from build123d import *

# Parameters (mm, degrees)
SKETCH004_R     = 64.00438
PAD_DEPTH       = 20
SKETCH006_R     = 4.5
POCKET_DEPTH    = 20
SKETCH005_R     = 4.5
POCKET001_DEPTH = 20
SKETCH007_W     = 10
SKETCH007_H     = 22
PAD001_DEPTH    = 70
SKETCH_W        = 16
SKETCH_H        = 40.7
POCKET002_DEPTH = 10
POCKET003_DEPTH = 20
SKETCH008_R     = 15
POCKET004_DEPTH = 20
SKETCH011_R     = 15
POCKET005_DEPTH = 20


with BuildPart() as part:
    # Sketch004 → Pad (new body)
    with BuildSketch(Plane.XY):
        Circle(SKETCH004_R)
    extrude(amount=PAD_DEPTH)

    # Sketch006 → Pocket (cut)
    with BuildSketch(Plane.XY):
        with Locations((20, 0)):
            Circle(SKETCH006_R)
    extrude(amount=POCKET_DEPTH, mode=Mode.SUBTRACT)

    # Sketch005 → Pocket001 (cut)
    with BuildSketch(Plane.XY):
        with Locations((-20, 0)):
            Circle(SKETCH005_R)
    extrude(amount=POCKET001_DEPTH, mode=Mode.SUBTRACT)

    # Sketch007 → Pad001 (join)
    with BuildSketch(Plane.XY):
        with Locations((-8, 0)):
            Rectangle(SKETCH007_W, SKETCH007_H)
    extrude(amount=-PAD001_DEPTH)

    # Sketch (on Face7 of Pad001) → Pocket002 (cut)
    with BuildSketch(Plane.YZ.offset(-3)):
        with Locations((0, -41.65)):
            Rectangle(SKETCH_W, SKETCH_H)
    extrude(amount=-POCKET002_DEPTH, mode=Mode.SUBTRACT)

    # Sketch001 → Pocket003 (cut)
    with BuildSketch(Plane.XY):
        with BuildLine():
            Line((-2.25, 1.75), (2.25, 1.75))
            ThreePointArc((2.25, -1.75), (2.850439, 0), (2.25, 1.75))
            Line((-2.25, -1.75), (2.25, -1.75))
            ThreePointArc((-2.25, 1.75), (-2.850439, 0), (-2.25, -1.75))
        make_face()
    extrude(amount=POCKET003_DEPTH, mode=Mode.SUBTRACT)

    # Sketch008 → Pocket004 (cut)
    with BuildSketch(Plane.XY):
        with Locations((0, 32)):
            Circle(SKETCH008_R)
    extrude(amount=POCKET004_DEPTH, mode=Mode.SUBTRACT)

    # Sketch011 → Pocket005 (cut)
    with BuildSketch(Plane.XY):
        with Locations((0, -32)):
            Circle(SKETCH011_R)
    extrude(amount=POCKET005_DEPTH, mode=Mode.SUBTRACT)


solid = part.part
Design review of the part built by this model. Coordinates are the model's own, in mm. A direction names the side the tool comes from. Coordinates: 2 decimals unless noted, no trailing zeros. Order: outer loops, then holes, each group sorted by start corner. A loop starts at its lowest first (then second) coordinate and runs counter-clockwise, first axis right, second up. Notation, with made-up numbers: (-4, -20.5) -> (1, -20.5) arc R35 cw to (1, 12.5) -> close; hole circle Ø2 at (75.25, 34.25). An arc over 180 degrees is marked (long way). One line per item, written item: value.
1) To check wall thickness, follow probe 1 along Y at (x, z) = (0, 14); probe 2 along Z at (x, y) = (-23, -24.5); probe 3 along Y at (x, z) = (-20, 10). State the ranges of each line that lie inside material, in increasing order. Write a range as [from, to].
Output values:
probe 1: y = [-64, -47], [-17, -1.75], [1.75, 17], [47, 64]
probe 2: z = [0, 20]
probe 3: y = [-60.8, -4.5], [4.5, 60.8]
2) We need section D-D, the plane y = -29. Give the boundary of the cut face in (x, z).
Output values:
outline: (-57.06, 0) -> (-14.7, 0) -> (-14.7, 20) -> (-57.06, 20) -> close; (14.7, 0) -> (57.06, 0) -> (57.06, 20) -> (14.7, 20) -> close
3) Draft analysis for pull direction X (two halves, no side actions). For faces 1 (the face through (-8, 0, -62)), 2 (the face through (-13, 0, -19)), 3 (the face through (0, -1.75, 10)), state which applies: +X half, -X half, draft (parallel to the pull), parting line (faces both ways), or undercut.
Output values:
face 1: draft
face 2: -X half
face 3: undercut
4) Clearance check with flat-ended pins moving along their axes: P1, Ø3, axis at x = -10, z = -46, coming from the -Y side; P2, Ø12, axis at x = -22.5, y = 36, coming from the -Z side; P3, Ø11, axis at y = 5, z = -32.5, coming from the +X side; P4, Ø24, axis at x = 0, y = 32, coming from the +Z side. State where each tip first meets the part, or that it passes through.
Output values:
P1: stops at y = -11
P2: stops at z = 0
P3: stops at x = -3
P4: passes through
5) We need section A-A, the plane z = -37.5. Give the boundary of the cut face in (x, y).
Output values:
outline: (-13, -11) -> (-3, -11) -> (-3, -8) -> (-13, -8) -> close; (-13, 8) -> (-3, 8) -> (-3, 11) -> (-13, 11) -> close
6) We need section B-B, the plane x = 0. Give the boundary of the cut face in (y, z).
Output values:
outline: (-64, 0) -> (-47, 0) -> (-47, 20) -> (-64, 20) -> close; (-17, 0) -> (-1.75, 0) -> (-1.75, 20) -> (-17, 20) -> close; (1.75, 0) -> (17, 0) -> (17, 20) -> (1.75, 20) -> close; (47, 0) -> (64, 0) -> (64, 20) -> (47, 20) -> close
7) We need section C-C, the plane y = 0. Give the boundary of the cut face in (x, z), then the cut area to 3 significant figures.
Output values:
outline: (-64, 0) -> (-24.5, 0) -> (-24.5, 20) -> (-64, 20) -> close; (-15.5, 0) -> (-13, 0) -> (-13, -21.3) -> (-3, -21.3) -> (-3, 0) -> (-2.85, 0) -> (-2.85, 20) -> (-15.5, 20) -> close; (-13, -70) -> (-3, -70) -> (-3, -62) -> (-13, -62) -> close; (2.85, 0) -> (15.5, 0) -> (15.5, 20) -> (2.85, 20) -> close; (24.5, 0) -> (64, 0) -> (64, 20) -> (24.5, 20) -> close
area: 2,380 mm2
8) Machinability: for faces 4 (the face through (-3, 0, -19)), 5 (the face through (2.85, -0.03, 9.86)), 6 (the face through (-8, -11, -35)), 7 (the face through (-8, -8, -42)), 8 (the face through (-8, 11, -35)), which of the approach directions +Z, -Z, +X, -X, +Y, -Y give a long, thin tool a straight path to every point of the face, cutting with its end or side? Answer none if there is none.
Output values:
face 4: -Z, +X, +Y, -Y
face 5: +Z, -Z
face 6: -Z, +X, -X, -Y
face 7: +X, -X
face 8: -Z, +X, -X, +Y
